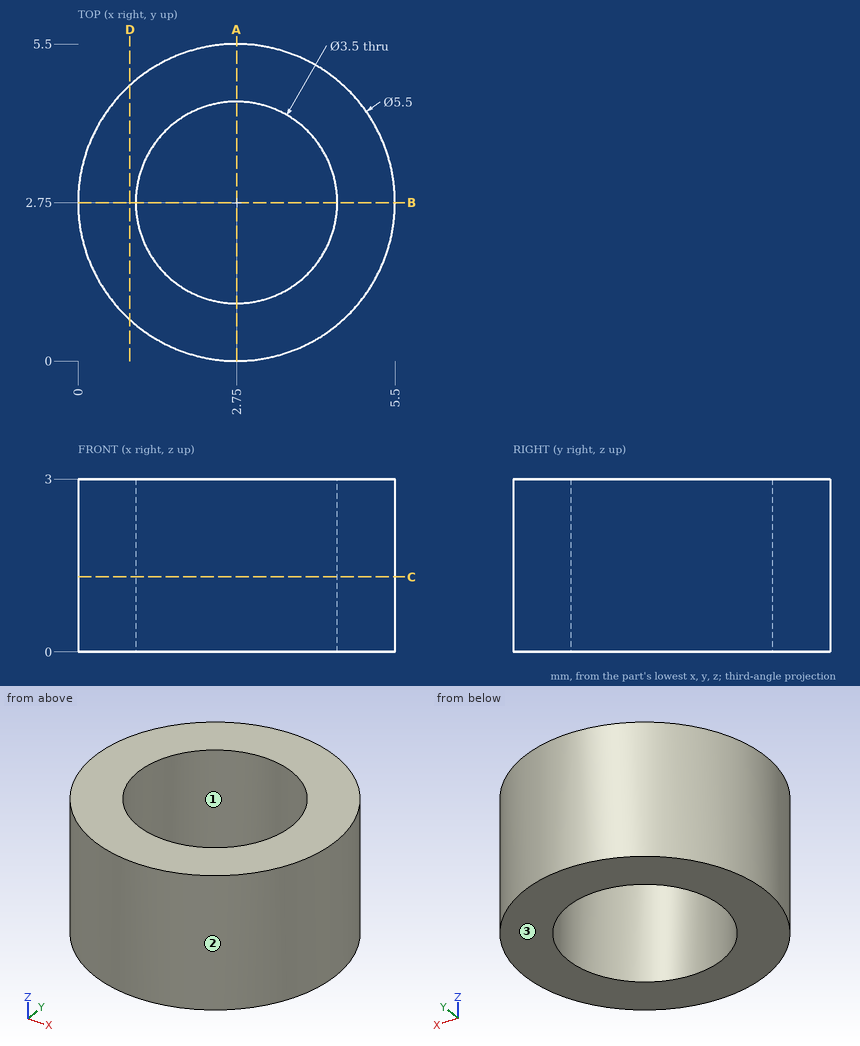
Verification items for this drawing (mm, ordinates from the low corner). Give positions to 0.01 mm unless a question says otherwise; leave off trailing zeros. Loops run counter-clockwise (first coordinate to the right, second up) from the corner with the lowest first, then second, coordinate; pieces in that order, holes last. Notation, with made-up numbers: M 52.25,83 L 57.25,83 A20 cw 57.25,115 Z; hole C -23,58 d2. An arc over 180 degrees is marked long. Answer as a JSON object with one key per item and string values. Group by question number.
Item 1: Sectioned sample at C-C on z = 1.3. Record the boundary of the cut face in (x, y).
Item 2: Material ranges on L1, parallel to Y at x = 2.75, z = 1.35; L2, parallel to X at y = 1.35, z = 2.15; L3, parallel to Y at x = 3.8, z = 2.85, recorded low to high.
Item 3: Mould release check, pull along X, two halves, no side actions. Record for the marked faces 1, 2 and 3: pulls with the +X half, pulls with the -X half, needs draft (parallel to the pull), parting line crosses it, or undercut.
Item 4: Sectioned sample at D-D on x = 0.9. Record the boundary of the cut face in (y, z), plus the area to 3 significant figures.
Item 5: Sectioned sample at A-A on x = 2.75. Record the boundary of the cut face in (y, z).
Item 6: Gauge pin test, flat end, axial feed: pin 1 (1 mm diameter, centred on y = 2, z = 2, fed in from +X). Record the tip position at first contact, or that the pin passes through.
Findings below:
{
 "1": {"outline": "C 2.75,2.75 d5.5; hole C 2.75,2.75 d3.5"},
 "2": {"L1": "0 to 1, 4.5 to 5.5", "L2": "0.38 to 1.7, 3.8 to 5.12", "L3": "0.21 to 1.35, 4.15 to 5.29"},
 "3": {"face 1": "undercut", "face 2": "parting line crosses it", "face 3": "needs draft"},
 "4": {"outline": "M 0.72,0 L 4.78,0 L 4.78,3 L 0.72,3 Z", "area": "12.2 mm2"},
 "5": {"outline": "M 0,0 L 1,0 L 1,3 L 0,3 Z; M 4.5,0 L 5.5,0 L 5.5,3 L 4.5,3 Z"},
 "6": {"pin 1": "x = 5.49"}
}
